CAD build for the part. Positions are in the model's coordinates, mm. A direction names the side the tool comes from. Round coordinates to 2 decimals unless told otherwise and drop trailing zeros. Loops run counter-clockwise (first coordinate to the right, second up) from the corner with the lowest first, then second, coordinate; pieces in that order, holes last. Notation, with made-up numbers: (2.25, 61) - (36.25, 61) arc R15 cw to (36.25, 69) - close; hole circle Ø7 at (50.25, 39.5). An arc over 180 degrees is marked (long way). Use one line per item in the form item = value.
from build123d import *

# Parameters (mm, degrees)
SKETCH1_W           = 40
SKETCH1_H           = 105
SKETCH1_R           = 4.25
BOSS_EXTRUDE1_DEPTH = 3
CHAMFER1_SIZE       = 5


with BuildPart() as part:
    # Sketch1 → Boss-Extrude1 (new body, symmetric)
    with BuildSketch(Plane.XY):
        Rectangle(SKETCH1_W, SKETCH1_H)
        with Locations((9, -32.5)):
            Circle(SKETCH1_R, mode=Mode.SUBTRACT)
        with Locations((-9, -32.5)):
            Circle(SKETCH1_R, mode=Mode.SUBTRACT)
        with BuildLine():
            Line((9, 36.5), (9, 26.5))
            ThreePointArc((9, 26.5), (0, 17.5), (-9, 26.5))
            Line((-9, 26.5), (-9, 36.5))
            ThreePointArc((-9, 36.5), (0, 45.5), (9, 36.5))
        make_face(mode=Mode.SUBTRACT)
    extrude(amount=BOSS_EXTRUDE1_DEPTH, both=True)

    # Chamfer1
    chamfer1_edges = [part.edges().sort_by_distance(p)[0] for p in [
        (-20, 52.5, 0),
        (20, 52.5, 0),
    ]]
    chamfer(chamfer1_edges, length=CHAMFER1_SIZE)


solid = part.part
1) Slice it at B-B (x = 0). Write the cut outline in (y, z), plus the area to 3 significant figures.
Report:
outline = (-52.5, -3) - (17.5, -3) - (17.5, 3) - (-52.5, 3) - close; (45.5, -3) - (52.5, -3) - (52.5, 3) - (45.5, 3) - close
area = 462 mm^2
2) Slice it at C-C (z = -0.1). Write the cut outline in (x, y).
Report:
outline = (-20, -52.5) - (20, -52.5) - (20, 47.5) - (15, 52.5) - (-15, 52.5) - (-20, 47.5) - close; hole circle Ø8.5 at (-9, -32.5); hole (-9, 26.5) arc R9 ccw to (9, 26.5) - (9, 36.5) arc R9 ccw to (-9, 36.5) - close; hole circle Ø8.5 at (9, -32.5)
3) Two-plate mould, pull along X, no slides. Class faces 3 (the flat face through (17.5, 50, 0)), 4 (the cylindrical face through (-12.37, -35.09, -0.04)), 5 (the flat face through (-17.5, 50, 0)), 6 (the flat face through (0, -52.5, 0)): +X half, -X half, draft (parallel to the pull), parting line (faces both ways), or undercut.
Report:
face_3 = +X half
face_4 = undercut
face_5 = -X half
face_6 = draft
4) Drill centre lines: probe 1 along X at (y, z) = (34, 2.15); probe 2 along Y at (x, z) = (-8, -2.3); probe 3 along Y at (x, z) = (9.5, -2.1). Where is each one in solid material? Low to high.
Report:
probe_1 = -20 to -9, 9 to 20
probe_2 = -52.5 to -36.63, -28.37 to 22.38, 40.62 to 52.5
probe_3 = -52.5 to -36.72, -28.28 to 52.5
5) Slice it at A-A (y = -32.5). Write the cut outline in (x, z).
Report:
outline = (-20, -3) - (-13.25, -3) - (-13.25, 3) - (-20, 3) - close; (-4.75, -3) - (4.75, -3) - (4.75, 3) - (-4.75, 3) - close; (13.25, -3) - (20, -3) - (20, 3) - (13.25, 3) - close
6) Slice it at D-D (y = 44). Write the cut outline in (x, z), plus the area to 3 significant figures.
Report:
outline = (-20, -3) - (-4.97, -3) - (-4.97, 3) - (-20, 3) - close; (4.97, -3) - (20, -3) - (20, 3) - (4.97, 3) - close
area = 180 mm^2
7) Tool access for faces 1 (the flat face through (-9, 31, 0)), 2 (the flat face through (20, -3, 0)): list every direction of +Z, -Z, +X, -X, +Y, -Y with a clear straight run to the whole face (end or side of a thin tool).
Report:
face_1 = +Z, -Z
face_2 = +Z, -Z, +X, +Y, -Y
8) Flat gauge pin, fed straight in: pin 1 (11 mm diameter, centred on x = 9, y = -32.5, fed in from -Z). Where does the tip first touch, or does it go through?
Report:
pin_1 = -3
